```python
from build123d import *

# Parameters (mm, degrees)
BASE_FLANGE1_DEPTH  = 80
SKETCH6_R           = 2.125
CUT_EXTRUDE1_DEPTH  = 275.800838609
FILLET1_R           = 5
BOSS_EXTRUDE1_DEPTH = 2.06
FILLET2_R           = 10
CUT_EXTRUDE2_DEPTH  = 10


# Read off the part's stored shape, not the designer's step: Base-Flange1
with BuildPart() as part:
    # Base-Flange1 outline → Base-Flange1 (new body)
    with BuildSketch(Plane(origin=(0, 0, 0), x_dir=(1, 0, 0), z_dir=(0, 1, 0))):
        with BuildLine():
            Line((-130, -3.076), (-130, -15))
            Line((-130, -15), (-127.94, -15))
            Line((-127.94, -15), (-127.94, -3.076))
            ThreePointArc((-127.94, -3.076), (-127.64242049, -2.35757951), (-126.924, -2.06))
            Line((-126.924, -2.06), (129.394, -2.06))
            ThreePointArc((129.394, -2.06), (130.11242049, -2.35757951), (130.41, -3.076))
            Line((130.41, -3.076), (130.41, -15))
            Line((130.41, -15), (132.47, -15))
            Line((132.47, -15), (132.47, -3.076))
            ThreePointArc((132.47, -3.076), (131.569060459, -0.900939541), (129.394, 0))
            Line((129.394, 0), (-126.924, 0))
            ThreePointArc((-126.924, 0), (-129.099060459, -0.900939541), (-130, -3.076))
        make_face()
    extrude(amount=BASE_FLANGE1_DEPTH)

    # Sketch6 → Cut-Extrude1 (cut, through all)
    with BuildSketch(Plane.ZY.offset(130)):
        with Locations((9.038, 70)):
            Circle(SKETCH6_R)
        with Locations((9.038, 10)):
            Circle(SKETCH6_R)
    extrude(amount=-CUT_EXTRUDE1_DEPTH, mode=Mode.SUBTRACT)

    # Fillet1
    fillet1_edges = [part.edges().sort_by_distance(p)[0] for p in [
        (131.44, 0, 15),
        (-128.97, 0, 15),
        (131.44, 80, 15),
        (-128.97, 80, 15),
    ]]
    fillet(fillet1_edges, radius=FILLET1_R)

    # Sketch7 → Boss-Extrude1 (add)
    with BuildSketch(Plane.XY.offset(2.06)):
        Polygon((-100, 0), (-80, -20), (80, -20), (100, 0), align=None)
    extrude(amount=-BOSS_EXTRUDE1_DEPTH)

    # Fillet2
    fillet2_edges = [part.edges().sort_by_distance(p)[0] for p in [
        (-100, 0, 1.03),
        (100, 0, 1.03),
        (80, -20, 1.03),
        (-80, -20, 1.03),
    ]]
    fillet(fillet2_edges, radius=FILLET2_R)

    # Sketch8 → Cut-Extrude2 (cut)
    with BuildSketch(Plane.XY.offset(2.06)):
        with BuildLine():
            Line((-96.924, 72), (-21.924, 72))
            ThreePointArc((-21.924, 72), (-19.924, 70), (-21.924, 68))
            Line((-21.924, 68), (-96.924, 68))
            ThreePointArc((-96.924, 68), (-98.924, 70), (-96.924, 72))
        make_face()
        with BuildLine():
            Line((-96.924, 58.66), (-21.924, 58.66))
            ThreePointArc((-21.924, 58.66), (-19.924, 56.66), (-21.924, 54.66))
            Line((-21.924, 54.66), (-96.924, 54.66))
            ThreePointArc((-96.924, 54.66), (-98.924, 56.66), (-96.924, 58.66))
        make_face()
        with BuildLine():
            Line((-96.924, 45.32), (-21.924, 45.32))
            ThreePointArc((-21.924, 45.32), (-19.924, 43.32), (-21.924, 41.32))
            Line((-21.924, 41.32), (-96.924, 41.32))
            ThreePointArc((-96.924, 41.32), (-98.924, 43.32), (-96.924, 45.32))
        make_face()
        with BuildLine():
            Line((-96.924, 31.98), (-21.924, 31.98))
            ThreePointArc((-21.924, 31.98), (-19.924, 29.98), (-21.924, 27.98))
            Line((-21.924, 27.98), (-96.924, 27.98))
            ThreePointArc((-96.924, 27.98), (-98.924, 29.98), (-96.924, 31.98))
        make_face()
        with BuildLine():
            Line((-96.924, 18.64), (-21.924, 18.64))
            ThreePointArc((-21.924, 18.64), (-19.924, 16.64), (-21.924, 14.64))
            Line((-21.924, 14.64), (-96.924, 14.64))
            ThreePointArc((-96.924, 14.64), (-98.924, 16.64), (-96.924, 18.64))
        make_face()
        with BuildLine():
            Line((96.924, 72), (21.924, 72))
            ThreePointArc((21.924, 72), (19.924, 70), (21.924, 68))
            Line((21.924, 68), (96.924, 68))
            ThreePointArc((96.924, 68), (98.924, 70), (96.924, 72))
        make_face()
        with BuildLine():
            Line((96.924, 58.66), (21.924, 58.66))
            ThreePointArc((21.924, 58.66), (19.924, 56.66), (21.924, 54.66))
            Line((21.924, 54.66), (96.924, 54.66))
            ThreePointArc((96.924, 54.66), (98.924, 56.66), (96.924, 58.66))
        make_face()
        with BuildLine():
            Line((96.924, 45.32), (21.924, 45.32))
            ThreePointArc((21.924, 45.32), (19.924, 43.32), (21.924, 41.32))
            Line((21.924, 41.32), (96.924, 41.32))
            ThreePointArc((96.924, 41.32), (98.924, 43.32), (96.924, 45.32))
        make_face()
        with BuildLine():
            Line((96.924, 31.98), (21.924, 31.98))
            ThreePointArc((21.924, 31.98), (19.924, 29.98), (21.924, 27.98))
            Line((21.924, 27.98), (96.924, 27.98))
            ThreePointArc((96.924, 27.98), (98.924, 29.98), (96.924, 31.98))
        make_face()
        with BuildLine():
            Line((96.924, 18.64), (21.924, 18.64))
            ThreePointArc((21.924, 18.64), (19.924, 16.64), (21.924, 14.64))
            Line((21.924, 14.64), (96.924, 14.64))
            ThreePointArc((96.924, 14.64), (98.924, 16.64), (96.924, 18.64))
        make_face()
    extrude(amount=-CUT_EXTRUDE2_DEPTH, mode=Mode.SUBTRACT)


solid = part.part
```
Design review of the part built by this model. Coordinates are the model's own, in mm. A direction names the side the tool comes from. Coordinates: 2 decimals unless noted, no trailing zeros. Loops run counter-clockwise (first coordinate to the right, second up) from the corner with the lowest first, then second, coordinate; pieces in that order, holes last. Notation, with made-up numbers: (59, 85) -> (106, 85) arc R16 cw to (106, 108) -> close; hole circle Ø10 at (4.25, -16). An arc over 180 degrees is marked (long way). Answer as a JSON object with one key per item and string values.
Q1. Take a section at A-A on x = -32.5. Give the boundary of the cut face in (y, z).
Answer block:
{"outline": "(-20, 0) -> (14.64, 0) -> (14.64, 2.06) -> (-20, 2.06) -> close; (18.64, 0) -> (27.98, 0) -> (27.98, 2.06) -> (18.64, 2.06) -> close; (31.98, 0) -> (41.32, 0) -> (41.32, 2.06) -> (31.98, 2.06) -> close; (45.32, 0) -> (54.66, 0) -> (54.66, 2.06) -> (45.32, 2.06) -> close; (58.66, 0) -> (68, 0) -> (68, 2.06) -> (58.66, 2.06) -> close; (72, 0) -> (80, 0) -> (80, 2.06) -> (72, 2.06) -> close"}
Q2. To check wall thickness, follow L1, parallel to Y at x = -24, z = 1; L2, parallel to X at y = 33.5, z = 6; L3, parallel to Z at x = 96.5, y = 40.5. State the ranges of each line that lie inside material, in increasing order.
Answer block:
{"L1": "y = -20 to 14.64, 18.64 to 27.98, 31.98 to 41.32, 45.32 to 54.66, 58.66 to 68, 72 to 80", "L2": "x = -130 to -127.94, 130.41 to 132.47", "L3": "z = 0 to 2.06"}
Q3. The part is to be moulded in two halves that separate along Y. For faces 5 (the flat face through (132.47, 39, 9)), 6 (the cylindrical face through (131.426, 9.186, 11.001)), 7 (the flat face through (90, -10, 1)), 8 (the cylindrical face through (-128.984, 72.107, 8.761)), say which applies: +Y half, -Y half, draft (parallel to the pull), parting line (faces both ways), or undercut.
Answer block:
{"face 5": "draft", "face 6": "undercut", "face 7": "-Y half", "face 8": "undercut"}
Q4. Tool access review of faces 1 (the flat face through (-119, 0, 1.6)), 2 (the flat face through (130.41, 39, 9)), 3 (the cylindrical face through (131.426, 72.107, 8.761)), 4 (the flat face through (120.3, 0, 1.6)): name each direction out of +Z, -Z, +X, -X, +Y, -Y from which nothing blocks a thin tool from reaching the whole face with its end or side.
Answer block:
{"face 1": "+Z, -Z, -X, -Y", "face 2": "+Z, +Y, -Y", "face 3": "+X, -X", "face 4": "+Z, -Z, +X, -Y"}
